from build123d import *

# Parameters (mm, degrees)
BOX022_W                   = 5.5
BOX022_H                   = 52
BOX022_DEPTH               = 8
PAD010_DEPTH               = 1.1
CHAMFER002_SIZE            = 1
CHAMFER002_PLACEMENT_ANGLE = 180
BOX021_W                   = 12.5
BOX021_H                   = 52
BOX021_DEPTH               = 4
BOX020_W                   = 16.5
BOX020_H                   = 56
BOX020_DEPTH               = 11


with BuildPart() as cube022:
    # Box022 → Box022 (new body)
    with BuildSketch(Plane(origin=(3.25, -9, -0.5), x_dir=(1, 0, 0), z_dir=(0, 0, 1))):
        with Locations((2.75, 26)):
            Rectangle(BOX022_W, BOX022_H)
    extrude(amount=BOX022_DEPTH)


with BuildPart() as chamfer002:
    # Sketch013 → Pad010 (new body)
    with BuildSketch(Plane.XY):
        Polygon((0, 20.777284), (-2.180816, 17), (2.180816, 17), align=None)
    extrude(amount=PAD010_DEPTH)

    # Chamfer002
    chamfer002_edges = [chamfer002.edges().sort_by_distance(p)[0] for p in [
        (-1.090408, 18.888642, 0),
        (0, 17, 0),
        (1.090408, 18.888642, 0),
    ]]
    chamfer(chamfer002_edges, length=CHAMFER002_SIZE)


with BuildPart() as chamfer002_1:
    # Chamfer002 placement: moved
    add(chamfer002.part.moved(Location((11.5, 12.5, 0.9))).rotate(Axis((11.5, 12.5, 0.9), (1, 0, 0)), CHAMFER002_PLACEMENT_ANGLE))


with BuildPart() as fusion012:
    # Box021 → Box021 (new body)
    with BuildSketch(Plane(origin=(-0.25, -9, 7.5), x_dir=(1, 0, 0), z_dir=(0, 0, 1))):
        with Locations((6.25, 26)):
            Rectangle(BOX021_W, BOX021_H)
    extrude(amount=BOX021_DEPTH)

    # Fusion012: union Cube022, Chamfer002
    add(cube022.part)
    add(chamfer002_1.part)


with BuildPart() as obj1:
    # Box020 → Box020 (new body)
    with BuildSketch(Plane(origin=(-2.25, -11, 0), x_dir=(1, 0, 0), z_dir=(0, 0, 1))):
        with Locations((8.25, 28)):
            Rectangle(BOX020_W, BOX020_H)
    extrude(amount=BOX020_DEPTH)

    # Cut023: cut Fusion012
    add(fusion012.part, mode=Mode.SUBTRACT)


solid = obj1.part
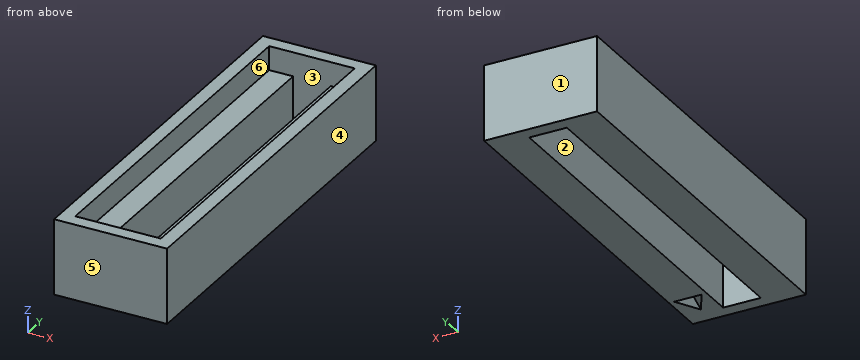
Could you check a few things on this model? Use its own coordinates, in mm. Face numbers are marked on the shaded views. A direction names the side the tool comes from. Give positions to 0.01 mm unless a question says otherwise; leave off trailing zeros. Order: outer loops, then holes, each group sorted by start corner. A loop starts at its lowest first (then second) coordinate and runs counter-clockwise, first axis right, second up.
Item 1: If we section it at D-D, the plane z = 2.75: Write out the boundary of the cut face in (x, y).
Item 2: For the marked faces 1, 2 and 3, which set-ups out of +Z, -Z, +X, -X, +Y, -Y let a thin tool reach every point of the face, with its end or its side?
Item 3: I need wall thicknesses on line 1 (X direction, y = 8, z = 9.25); line 2 (Y direction, x = 1.5, z = 9); line 3 (X direction, y = 34, z = 2.75). Which ranges of each line are inside material? Lowest first, please.
Item 4: If we section it at C-C, the plane y = 40: Write out the boundary of the cut face in (x, z), plus the area to 3 significant figures.
Item 5: If we mould it in two halves opening along Y, with no side actions, what happens to the marked faces 4, 5 and 6? For each: pulls with the +Y half, pulls with the -Y half, needs draft (parallel to the pull), parting line crosses it, or undercut.
Item 6: If we section it at B-B, the plane x = 8: Write out the boundary of the cut face in (y, z).
Item 7: If we section it at A-A, the plane z = 9: Write out the boundary of the cut face in (x, y).
Item 8: I'm going to push flat-ended pins straight in: pin 1 (0.6 mm diameter, centred on x = 11.5, y = -5.5, fed in from -Z); pin 2 (1 mm diameter, centred on x = 9, y = 36, fed in from +Z). Where does each tip first touch, or does it pass through?
Values:
1. outline: (-2.25, -11) - (14.25, -11) - (14.25, 45) - (-2.25, 45) - close; hole (3.25, -9) - (8.75, -9) - (8.75, 43) - (3.25, 43) - close
2. face 1: +Z, -Z, +X, -X, +Y
2. face 2: +Z, -Z
2. face 3: +Z
3. line 1: x = -2.25 to -0.25, 12.25 to 14.25
3. line 2: y = -11 to -9, 43 to 45
3. line 3: x = -2.25 to 3.25, 8.75 to 14.25
4. outline: (-2.25, 0) - (3.25, 0) - (3.25, 7.5) - (-0.25, 7.5) - (-0.25, 11) - (-2.25, 11) - close; (8.75, 0) - (14.25, 0) - (14.25, 11) - (12.25, 11) - (12.25, 7.5) - (8.75, 7.5) - close
4. area: 96.5 mm2
5. face 4: needs draft
5. face 5: pulls with the -Y half
5. face 6: undercut
6. outline: (-11, 0) - (-9, 0) - (-9, 11) - (-11, 11) - close; (43, 0) - (45, 0) - (45, 11) - (43, 11) - close
7. outline: (-2.25, -11) - (14.25, -11) - (14.25, 45) - (-2.25, 45) - close; hole (-0.25, -9) - (12.25, -9) - (12.25, 43) - (-0.25, 43) - close
8. pin 1: stops at z = 0.6
8. pin 2: stops at z = 7.5
